Autodesk Inventor part; units mm, degrees
ref_plane "YZ Plane" through (0, 0, 0) normal (1, 0, 0) x (0, 1, 0)
ref_plane "XZ Plane" through (0, 0, 0) normal (0, 1, 0) x (-1, 0, 0)
ref_plane "XY Plane" through (0, 0, 0) normal (0, 0, 1) x (1, 0, 0)
sketch "Sketch1" plane through (0, 0, 0) normal (0, 0, 1) x (1, 0, 0)
  line L0 (-12.1708, 16.0073) -> (13.2292, 16.0073)
  line L1 (13.2292, 16.0073) -> (13.2292, -34.7927)
  line L2 (13.2292, -34.7927) -> (-12.1708, -34.7927)
  line L3 (-12.1708, -34.7927) -> (-12.1708, 16.0073)
  line L4 (11.9592, 14.7373) -> (-10.9008, 14.7373)
  line L5 (-10.9008, 14.7373) -> (-10.9008, -33.5227)
  line L6 (-10.9008, -33.5227) -> (11.9592, -33.5227)
  line L7 (11.9592, -33.5227) -> (11.9592, 14.7373)
  point P0 (0, 0)
  dimension "d0" = 25.4
  dimension "d1" = 50.8
  dimension "d2" = 1.27
extrude "Extrusion1" add sketch "Sketch1" along normal blind 609.6
sketch "Sketch2" plane through (-12.1708, 16.0073, 0) normal (0, 1, 0) x (1, 0, 0)
  circle A0 centre (12.7, -12.7) radius 1.7272
  line L0 (25.4, 0) -> (0, 0)
  line L1 (0, 0) -> (0, -609.6)
  point P0 (12.1708, 0)
  dimension "d5" = 3.4544
  dimension "d6" = 12.7
  dimension "d7" = 12.7
extrude "Extrusion2" cut sketch "Sketch2" against normal through all
pattern_linear "Rectangular Pattern1" count 61 spacing 25.4 along (0, 0, 1) of "Extrusion2"
sketch "Sketch3" plane through (13.2292, -34.7927, 0) normal (1, 0, 0) x (0, 0, -1)
  circle A0 centre (-495.3, 25.4) radius 14.2875
  line L0 (-609.6, 0) -> (-609.6, 50.8)
  line L1 (0, 0) -> (-609.6, 0)
  circle A1 centre (-279.4, 25.4) radius 14.2875
  circle A2 centre (-101.6, 25.4) radius 14.2875
  point P0 (0, 34.7927)
  point P1 (-609.6, 25.4)
  dimension "d15" = 28.575
  dimension "d16" = 114.3
  dimension "d17" = 25.4
  dimension "d18" = 28.575
  dimension "d19" = 330.2
  dimension "d20" = 28.575
  dimension "d21" = 177.8
  dimension "d22" = 25.4
  dimension "d23" = 25.4
extrude "Extrusion3" cut sketch "Sketch3" against normal blind 214.3125
equation "\"d3\" = d13"
equation "\"d10\" = d14"
equation "\"d13\" = 609.6"
equation "\"d14\" = d13"
properties part number "intake versa"
The model under review builds one solid part; all positions refer to its coordinate system, in mm. A direction names the side the tool comes from. Round coordinates to 2 decimals unless told otherwise and drop trailing zeros. Loops run counter-clockwise (first coordinate to the right, second up) from the corner with the lowest first, then second, coordinate; pieces in that order, holes last. Notation, with made-up numbers: (70.5, 28.5) -> (84.5, 28.5) arc R14 ccw to (84.5, 34.5) -> close; hole circle Ø1 at (33.25, 48). An arc over 180 degrees is marked (long way). Answer as a JSON object with one key per item and string values. Group by question number.
1) For line 1 (X direction, y = -16, z = 197); line 2 (Y direction, x = -8.5, z = 393.5); line 3 (Y direction, x = 13, z = 279.4), list the stretches that pass through material, from the lowest coordinate up. Write a range as [from, to].
2) We need section B-B on x = 7.75. Write out the cut boundary in (y, z).
3) For faces 1 (the face through (0, -33.523, 301)), 2 (the face through (13.229, -9, 301)), list the 3-axis set-ups (+Z, -Z, +X, -X, +Y, -Y) from which the entire face can be reached by the end or side of a thin tool; tool diameter is ignored.
4) We need section A-A on z = 48. Write out the cut boundary in (x, y).
5) Mouldability with a two-part tool opening along Y and no side actions: class faces 3 (the face through (-12.171, -10, 301)), 4 (the face through (1, 14.737, 301)), 5 (the face through (0, 16.007, 301)) as released by +Y, released by -Y, zero draft, split by the parting line, or undercut.
Result set:
{
 "1": {"line 1": "[-12.17, -10.9], [11.96, 13.23]", "line 2": "[-34.79, -33.52], [14.74, 16.01]", "line 3": "[-34.79, -23.68], [4.89, 16.01]"},
 "2": {"outline": "(-34.79, 0) -> (-33.52, 0) -> (-33.52, 609.6) -> (-34.79, 609.6) -> close; (14.74, 0) -> (16.01, 0) -> (16.01, 609.6) -> (14.74, 609.6) -> close"},
 "3": {"face 1": "+Z, -Z", "face 2": "+Z, -Z, +X, +Y, -Y"},
 "4": {"outline": "(-12.17, -34.79) -> (13.23, -34.79) -> (13.23, 16.01) -> (-12.17, 16.01) -> close; hole (-10.9, -33.52) -> (11.96, -33.52) -> (11.96, 14.74) -> (-10.9, 14.74) -> close"},
 "5": {"face 3": "zero draft", "face 4": "undercut", "face 5": "released by +Y"}
}
